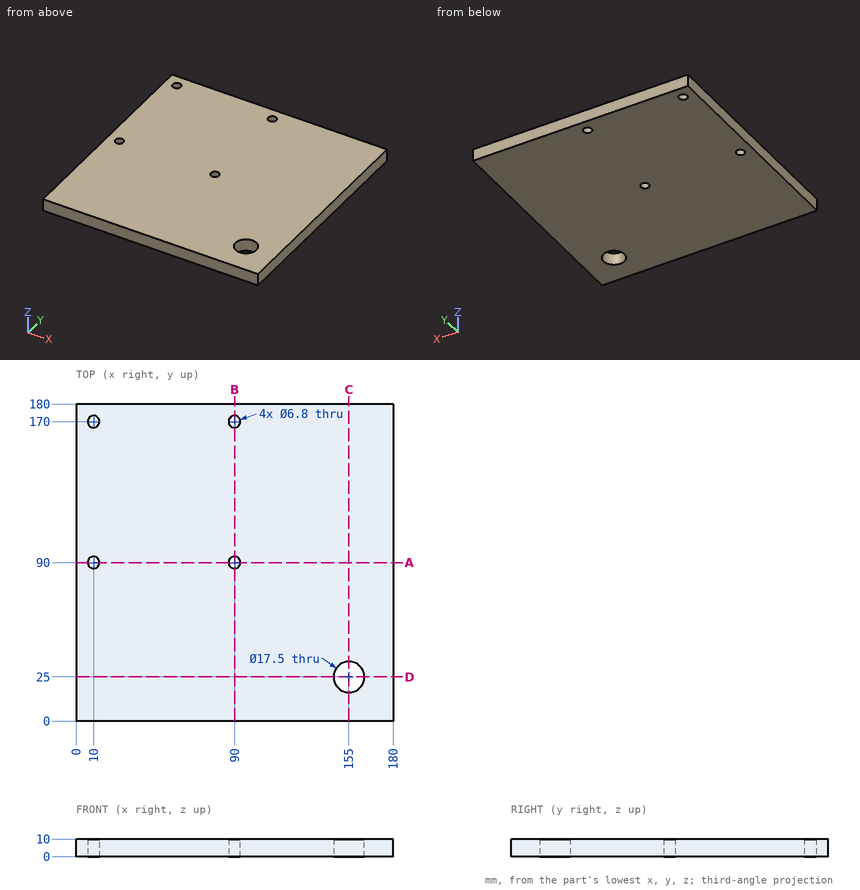
Print and shaded views of the part. All mm, measured from the part's lowest x, y and z. Round coordinates to 2 decimals unless told otherwise and drop trailing zeros. Order: outer loops, then holes, each group sorted by start corner. A loop starts at its lowest first (then second) coordinate and runs counter-clockwise, first axis right, second up. Notation, with made-up numbers: (-8, 38.25) - (8, 38.25) arc R26 ccw to (8, 60.25) - close; hole circle Ø9 at (57.25, 7.25). An arc over 180 degrees is marked (long way). Use a Markdown table: item, result.
1) Saw through at D-D on y = 25. Write the cut outline in (x, z), and give its area (4 significant figures).
Recorded:
| item | result |
|---|---|
| outline | (0, 0) - (146.25, 0) - (146.25, 10) - (0, 10) - close; (163.75, 0) - (180, 0) - (180, 10) - (163.75, 10) - close |
| area | 1,625 mm² |
2) Saw through at B-B on x = 90. Write the cut outline in (y, z).
Recorded:
| item | result |
|---|---|
| outline | (0, 0) - (86.6, 0) - (86.6, 10) - (0, 10) - close; (93.4, 0) - (166.6, 0) - (166.6, 10) - (93.4, 10) - close; (173.4, 0) - (180, 0) - (180, 10) - (173.4, 10) - close |
3) Flat gauge pins, fed straight in: pin 1 Ø5.5 at (x, y) = (90, 170) entering from +Z; pin 2 Ø6 at (x, y) = (30, 119.5) entering from -Z. Where does each tip first touch, or does it go through?
Recorded:
| item | result |
|---|---|
| pin 1 | passes through |
| pin 2 | stops at z = 0 |
4) Saw through at C-C on x = 155. Write the cut outline in (y, z).
Recorded:
| item | result |
|---|---|
| outline | (0, 0) - (16.25, 0) - (16.25, 10) - (0, 10) - close; (33.75, 0) - (180, 0) - (180, 10) - (33.75, 10) - close |
5) Wall check: L1, parallel to Y at x = 90, z = 4.25; L2, parallel to X at y = 90, z = 6; L3, parallel to Y at x = 155, z = 4. Give the ranges that are in metal, low to high.
Recorded:
| item | result |
|---|---|
| L1 | y = 0 to 86.6, 93.4 to 166.6, 173.4 to 180 |
| L2 | x = 0 to 6.6, 13.4 to 86.6, 93.4 to 180 |
| L3 | y = 0 to 16.25, 33.75 to 180 |
6) Saw through at A-A on y = 90. Write the cut outline in (x, z).
Recorded:
| item | result |
|---|---|
| outline | (0, 0) - (6.6, 0) - (6.6, 10) - (0, 10) - close; (13.4, 0) - (86.6, 0) - (86.6, 10) - (13.4, 10) - close; (93.4, 0) - (180, 0) - (180, 10) - (93.4, 10) - close |
